Geometry: final body of the model. Coordinates: model frame, mm. Round coordinates to 2 decimals unless told otherwise and drop trailing zeros. Order: outer loops, then holes, each group sorted by start corner. A loop starts at its lowest first (then second) coordinate and runs counter-clockwise, first axis right, second up. Notation, with made-up numbers: M -17.5,48 L 10.5,48 A15 cw 10.5,53 Z; hole C -34.5,11.25 d9. An arc over 180 degrees is marked long. Put each result on its own line as item: value. Start each with the question number.
1) Material intervals for probe 1 along Y at (x, z) = (257.5, 11.5); probe 2 along Z at (x, y) = (176, 160.5); probe 3 along X at (y, z) = (59, 6.75), sorted ascending. Write a range as [from, to].
2) First-contact query: P1, Ø6.5, axis at x = 109.5, y = 8.5, coming from the +Z side; P2, Ø1.9, axis at y = 165, z = 10.5, coming from the -X side; P3, Ø4, axis at y = 187, z = 7.5, coming from the -X side. Flat tips, straight axial feed; report the tip coordinate or a pass-through.
3) Section A-A, the plane x = 71. Return loops of the section in (y, z).
4) Section B-B, the plane z = 10.75. Return loops of the section in (x, y), then the cut area to 3 significant figures.
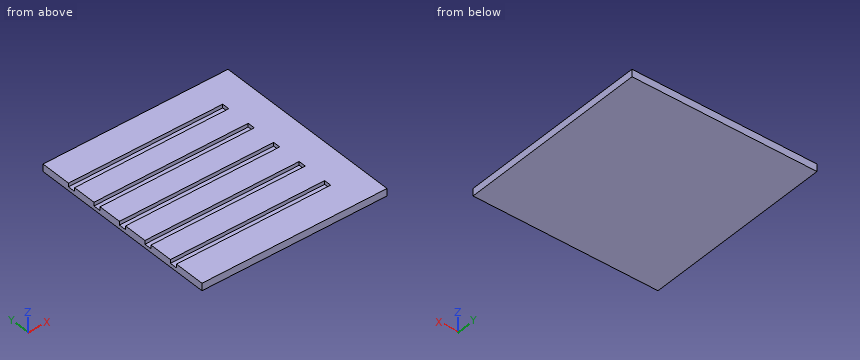
Autodesk Inventor part; units mm, degrees
ref_plane "YZ Plane" through (0, 0, 0) normal (1, 0, 0) x (0, 1, 0)
ref_plane "XZ Plane" through (0, 0, 0) normal (0, 1, 0) x (-1, 0, 0)
ref_plane "XY Plane" through (0, 0, 0) normal (0, 0, 1) x (1, 0, 0)
sketch "Sketch1" plane through (0, 0, 0) normal (0, 0, 1) x (1, 0, 0)
  line L0 (0, 0) -> (279.4, 0)
  line L1 (279.4, 0) -> (279.4, 279.4)
  line L2 (279.4, 279.4) -> (0, 279.4)
  line L3 (0, 279.4) -> (0, 0)
  dimension "d0" = 279.4
  dimension "d1" = 279.4
extrude "Extrusion1" add sketch "Sketch1" along normal blind 12.7
sketch "Sketch2" plane through (0, 0, 12.7) normal (0, 0, 1) x (1, 0, 0)
  line L0 (279.4, 0) -> (279.4, 279.4)
  line L1 (0, 0) -> (279.4, 0)
  line L2 (279.4, 0) -> (279.4, 12.7)
  line L3 (279.4, 12.7) -> (0, 12.7)
  line L4 (0, 12.7) -> (0, 0)
  line L5 (0, 279.4) -> (0, 0)
  line L6 (0, 53.34) -> (279.4, 53.34)
  line L7 (279.4, 53.34) -> (279.4, 66.04)
  line L8 (279.4, 66.04) -> (0, 66.04)
  line L9 (0, 66.04) -> (0, 53.34)
  line L10 (0, 106.68) -> (279.4, 106.68)
  line L11 (279.4, 106.68) -> (279.4, 119.38)
  line L12 (279.4, 119.38) -> (0, 119.38)
  line L13 (0, 119.38) -> (0, 106.68)
  line L14 (0, 160.02) -> (279.4, 160.02)
  line L15 (279.4, 160.02) -> (279.4, 172.72)
  line L16 (279.4, 172.72) -> (0, 172.72)
  line L17 (0, 172.72) -> (0, 160.02)
  line L18 (0, 213.36) -> (279.4, 213.36)
  line L19 (279.4, 213.36) -> (279.4, 226.06)
  line L20 (279.4, 226.06) -> (0, 226.06)
  line L21 (0, 226.06) -> (0, 213.36)
  point P0 (0, 66.04)
  point P1 (0, 119.38)
  point P2 (0, 172.72)
  point P3 (0, 226.06)
  dimension "d4" = 12.7
  dimension "d5" = 12.7
  dimension "d6" = 40.64
  dimension "d7" = 12.7
  dimension "d8" = 40.64
  dimension "d9" = 12.7
  dimension "d10" = 40.64
  dimension "d11" = 12.7
  dimension "d12" = 40.64
extrude "Extrusion2" cut sketch "Sketch2" against normal blind 6.35 contours L1 L4 L3 L0 | L6 L5 L8 L0 | L10 L5 L12 L0 | L14 L5 L16 L0 | L18 L5 L20 L0
sketch "Sketch3" plane through (279.4, 0, 0) normal (1, 0, 0) x (0, 0, -1)
  point P0 (0, 0)
sketch "Sketch4" plane through (279.4, 0, 0) normal (1, 0, 0) x (0, 0, -1)
  line L0 (-6.35, 106.68) -> (-12.7, 106.68)
  line L1 (-12.7, 66.04) -> (-12.7, 106.68)
  line L2 (-12.7, 66.04) -> (-6.35, 66.04)
  line L3 (-6.35, 66.04) -> (-6.35, 53.34)
  line L4 (-6.35, 53.34) -> (-12.7, 53.34)
  line L5 (-12.7, 12.7) -> (-12.7, 53.34)
  line L6 (-12.7, 12.7) -> (-6.35, 12.7)
  line L7 (-6.35, 12.7) -> (-6.35, 0)
  line L8 (0, 0) -> (-6.35, 0)
  line L9 (0, 0) -> (0, 279.4)
  line L10 (0, 279.4) -> (-12.7, 279.4)
  line L11 (-12.7, 226.06) -> (-12.7, 279.4)
  line L12 (-12.7, 226.06) -> (-6.35, 226.06)
  line L13 (-6.35, 226.06) -> (-6.35, 213.36)
  line L14 (-6.35, 213.36) -> (-12.7, 213.36)
  line L15 (-12.7, 172.72) -> (-12.7, 213.36)
  line L16 (-12.7, 172.72) -> (-6.35, 172.72)
  line L17 (-6.35, 172.72) -> (-6.35, 160.02)
  line L18 (-6.35, 160.02) -> (-12.7, 160.02)
  line L19 (-12.7, 119.38) -> (-12.7, 160.02)
  line L20 (-12.7, 119.38) -> (-6.35, 119.38)
  line L21 (-6.35, 119.38) -> (-6.35, 106.68)
  point P0 (0, 0)
extrude "Extrusion3" cut sketch "Sketch4" against normal blind 12.7
sketch "Sketch5" plane through (0, 0, 0) normal (0, -1, 0) x (1, 0, 0)
  line L0 (0, 0) -> (266.7, 0)
  line L1 (266.7, 12.7) -> (0, 12.7)
  line L2 (0, 0) -> (266.7, 0)
  line L3 (266.7, 0) -> (266.7, 12.7)
  line L4 (266.7, 12.7) -> (0, 12.7)
  line L5 (0, 12.7) -> (0, 0)
extrude "Extrusion4" add sketch "Sketch5" along normal blind 53.34
sketch "Sketch6" plane through (266.7, 0, 0) normal (1, 0, 0) x (0, 0, -1)
  line L0 (0, 279.4) -> (0, -53.34)
  line L1 (-12.7, 279.4) -> (-12.7, 226.06)
  line L2 (0, -53.34) -> (-12.7, -53.34)
  line L3 (-12.7, -53.34) -> (-12.7, 279.4)
  line L4 (-12.7, 279.4) -> (0, 279.4)
  line L5 (0, 279.4) -> (0, -53.34)
  point P0 (0, 0)
extrude "Extrusion5" add sketch "Sketch6" along normal blind 53.34
properties part number "FrntBck Plate"
Result sheet:
1. probe 1: y = [-53.34, 0], [12.7, 53.34], [66.04, 106.68], [119.38, 160.02], [172.72, 213.36], [226.06, 279.4]
1. probe 2: z = [0, 6.35]
1. probe 3: x = [266.7, 320.04]
2. P1: stops at z = 6.35
2. P2: stops at x = 266.7
2. P3: stops at x = 0
3. outline: M -53.34,0 L 279.4,0 L 279.4,12.7 L 226.06,12.7 L 226.06,6.35 L 213.36,6.35 L 213.36,12.7 L 172.72,12.7 L 172.72,6.35 L 160.02,6.35 L 160.02,12.7 L 119.38,12.7 L 119.38,6.35 L 106.68,6.35 L 106.68,12.7 L 66.04,12.7 L 66.04,6.35 L 53.34,6.35 L 53.34,12.7 L 12.7,12.7 L 12.7,6.35 L 0,6.35 L 0,12.7 L -53.34,12.7 Z
4. outline: M 0,-53.34 L 320.04,-53.34 L 320.04,279.4 L 0,279.4 L 0,226.06 L 266.7,226.06 L 266.7,213.36 L 0,213.36 L 0,172.72 L 266.7,172.72 L 266.7,160.02 L 0,160.02 L 0,119.38 L 266.7,119.38 L 266.7,106.68 L 0,106.68 L 0,66.04 L 266.7,66.04 L 266.7,53.34 L 0,53.34 L 0,12.7 L 266.7,12.7 L 266.7,0 L 0,0 Z
4. area: 89,600 mm2
